from build123d import *

# Parameters (mm, degrees)
SKETCH1_W           = 90
SKETCH1_H           = 132
BOSS_EXTRUDE1_DEPTH = 3
SKETCH7_W           = 90
SKETCH7_H           = 13
BOSS_EXTRUDE7_DEPTH = 3
SKETCH5_W           = 3
SKETCH5_H           = 15
BOSS_EXTRUDE5_DEPTH = 3
SKETCH6_W           = 40
SKETCH6_H           = 3
BOSS_EXTRUDE6_DEPTH = 3
SKETCH8_R           = 8.15
CUT_EXTRUDE1_DEPTH  = 3


with BuildPart() as part:
    # Sketch1 → Boss-Extrude1 (new body)
    with BuildSketch(Plane(origin=(0, 0, 0), x_dir=(1, 0, 0), z_dir=(0, 1, 0))):
        with Locations((45, 66)):
            Rectangle(SKETCH1_W, SKETCH1_H)
    extrude(amount=BOSS_EXTRUDE1_DEPTH)

    # Sketch7 → Boss-Extrude7 (add)
    with BuildSketch(Plane(origin=(0, 3, 0), x_dir=(1, 0, 0), z_dir=(0, 1, 0))):
        with Locations((45, 138.5)):
            Rectangle(SKETCH7_W, SKETCH7_H)
    extrude(amount=-BOSS_EXTRUDE7_DEPTH)

    # Sketch5 → Boss-Extrude5 (add)
    with BuildSketch(Plane(origin=(0, 3, 0), x_dir=(1, 0, 0), z_dir=(0, 1, 0))):
        with Locations((-1.5, 127.5)):
            Rectangle(SKETCH5_W, SKETCH5_H)
        with Locations((-1.5, 72.5)):
            Rectangle(SKETCH5_W, SKETCH5_H)
        with Locations((-1.5, 17.5)):
            Rectangle(SKETCH5_W, SKETCH5_H)
        with Locations((91.5, 127.5)):
            Rectangle(SKETCH5_W, SKETCH5_H)
        with Locations((91.5, 72.5)):
            Rectangle(SKETCH5_W, SKETCH5_H)
        with Locations((91.5, 17.5)):
            Rectangle(SKETCH5_W, SKETCH5_H)
    extrude(amount=-BOSS_EXTRUDE5_DEPTH)

    # Sketch6 → Boss-Extrude6 (add)
    with BuildSketch(Plane(origin=(0, 3, 0), x_dir=(1, 0, 0), z_dir=(0, 1, 0))):
        with Locations((45, 146.5)):
            Rectangle(SKETCH6_W, SKETCH6_H)
    extrude(amount=-BOSS_EXTRUDE6_DEPTH)

    # Sketch8 → Cut-Extrude1 (cut)
    with BuildSketch(Plane(origin=(0, 3, 0), x_dir=(1, 0, 0), z_dir=(0, 1, 0))):
        with Locations((32.31, 72.5)):
            Circle(SKETCH8_R)
        with Locations((57.69, 72.5)):
            Circle(SKETCH8_R)
    extrude(amount=-CUT_EXTRUDE1_DEPTH, mode=Mode.SUBTRACT)


solid = part.part
Geometry: final body of the model. Coordinates: model frame, mm. A direction names the side the tool comes from. Round coordinates to 2 decimals unless told otherwise and drop trailing zeros. Order: outer loops, then holes, each group sorted by start corner. A loop starts at its lowest first (then second) coordinate and runs counter-clockwise, first axis right, second up. Notation, with made-up numbers: (85, 42.25) - (130, 42.25) arc R28 ccw to (130, 67.25) - close; hole circle Ø9 at (18, 49). An arc over 180 degrees is marked (long way). Write each question's results on one line, items separated by ' | '.
Item 1: Reachability of faces 1 (the flat face through (90, 2, -45)), 2 (the flat face through (-2, 2, -120)), 3 (the flat face through (65, 2, -146)), 4 (the flat face through (12, 2, -145)), 5 (the flat face through (0, 2, -5)) from +Z, -Z, +X, -X, +Y, -Y: full face, straight path, thin tool, end or side. Return the list, or none.
Completed:
face 1: +X, +Y, -Y | face 2: -X, +Y, -Y | face 3: -Z, +X, +Y, -Y | face 4: -Z, -X, +Y, -Y | face 5: +Z, -X, +Y, -Y
Item 2: Material intervals for line 1 along X through (y, z) = (0.6, -72.5); line 2 along Z through (x, y) = (57.69, 1.1); line 3 along X through (y, z) = (0.3, -67.5), sorted ascending. Write a range as [from, to].
Completed:
line 1: [-3, 24.16], [40.46, 49.54], [65.84, 93] | line 2: [-148, -80.65], [-64.35, 0] | line 3: [-3, 25.87], [38.75, 51.25], [64.13, 93]
Item 3: Section D-D, the plane z = -56.5. Return the cut outline in (x, y), and give its area (3 significant figures).
Completed:
outline: (0, 0) - (90, 0) - (90, 3) - (0, 3) - close | area: 270 mm^2
Item 4: Section B-B, the plane y = 2.35. State how many separate pieces and enclosed holes the cut face has, and give its area (3 significant figures).
Completed:
separate pieces: 1 | enclosed holes: 2 | area: 13,000 mm^2
Item 5: First-contact query: pin 1 Ø1.5 at (y, z) = (2, -36) entering from -X; pin 2 Ø1.5 at (y, z) = (1, -147) entering from -X; pin 3 Ø1.5 at (x, y) = (9.5, 2) entering from -Z. Flat tips, straight axial feed; report the tip coordinate or a pass-through.
Completed:
pin 1: x = 0 | pin 2: x = 25 | pin 3: z = -145
Item 6: Section C-C, the plane x = 57.69. Return the cut outline in (y, z).
Completed:
outline: (0, -148) - (3, -148) - (3, -80.65) - (0, -80.65) - close; (0, -64.35) - (3, -64.35) - (3, 0) - (0, 0) - close
Item 7: Section A-A, the plane z = -72.5. Return the cut outline in (x, y).
Completed:
outline: (-3, 0) - (24.16, 0) - (24.16, 3) - (-3, 3) - close; (40.46, 0) - (49.54, 0) - (49.54, 3) - (40.46, 3) - close; (65.84, 0) - (93, 0) - (93, 3) - (65.84, 3) - close
Item 8: Mould query, pull axis Z, two halves, no side actions, for faces 6 (the flat face through (-2, 2, -10)), 7 (the flat face through (93, 2, -72)), 8 (the flat face through (91, 2, -120)). Classes: pulls with the +Z half, pulls with the -Z half, needs draft (parallel to the pull), parting line crosses it, or undercut.
Completed:
face 6: pulls with the +Z half | face 7: needs draft | face 8: undercut
